Verification items for the finished model (mm, model axes). Round coordinates to 2 decimals unless told otherwise and drop trailing zeros. Write each loop counter-clockwise with the first axis right and the second up, starting at its lowest first coordinate (ties: lowest second). Pieces come first, ordered by that corner, then holes. Notation, with made-up numbers: (22.25, 75.5) - (77.25, 75.5) arc R26 cw to (77.25, 112.5) - close; hole circle Ø7 at (45.25, -25). An arc over 180 degrees is marked (long way). Answer as a JSON object with one key per item and string values.
```python
from build123d import *

# Parameters (mm, degrees)
F0_R     = 7.5
F1_DEPTH = 11


# Not quite as in the source:
# - a feature of the source that left no trace in its solid (it failed there, or was rolled back) is left out


with BuildPart() as f1:
    # F0 (on Front) → F1 (new body)
    with BuildSketch(Plane.XZ):
        with BuildLine():
            ThreePointArc((6.9961100303, 104.7666666667), (0, 98), (-6.9961100303, 104.7666666667))
            ThreePointArc((-6.9961100303, 104.7666666667), (-105, 0), (-6.9961100303, -104.7666666667))
            ThreePointArc((-6.9961100303, -104.7666666667), (0, -98), (6.9961100303, -104.7666666667))
            ThreePointArc((6.9961100303, -104.7666666667), (105, 0), (6.9961100303, 104.7666666667))
        make_face()
        with Locations((-59.54553545, -60.6574744609)):
            Circle(F0_R, mode=Mode.SUBTRACT)
        with Locations((-22.7581460876, -81.8966836121)):
            Circle(F0_R, mode=Mode.SUBTRACT)
        with Locations((-82.3036815375, -21.2392091511)):
            Circle(F0_R, mode=Mode.SUBTRACT)
        with Locations((22.7581460876, -81.8966836121)):
            Circle(F0_R, mode=Mode.SUBTRACT)
        with Locations((59.54553545, -60.6574744609)):
            Circle(F0_R, mode=Mode.SUBTRACT)
        with Locations((82.3036815375, -21.2392091511)):
            Circle(F0_R, mode=Mode.SUBTRACT)
        with Locations((-82.3036815375, 21.2392091511)):
            Circle(F0_R, mode=Mode.SUBTRACT)
        with Locations((-59.54553545, 60.6574744609)):
            Circle(F0_R, mode=Mode.SUBTRACT)
        with BuildLine():
            ThreePointArc((-15.2581460876, 81.8966836121), (-16.7869427812, 77.3585418036), (-20.750074374, 74.6705056463))
            ThreePointArc((-20.750074374, 74.6705056463), (-28.729349394, 86.4348254206), (-15.2581460876, 81.8966836121))
        make_face(mode=Mode.SUBTRACT)
        with BuildLine():
            ThreePointArc((10.3081014632, 37.0943802243), (30.6521769727, 23.2957946169), (38.5, 0))
            ThreePointArc((38.5, 0), (-23.2957946169, -30.6521769727), (-10.3081014632, 37.0943802243))
            ThreePointArc((-10.3081014632, 37.0943802243), (0, 38.5), (10.3081014632, 37.0943802243))
        make_face(mode=Mode.SUBTRACT)
        with Locations((82.3036815375, 21.2392091511)):
            Circle(F0_R, mode=Mode.SUBTRACT)
        with BuildLine():
            ThreePointArc((30.2581460876, 81.8966836121), (27.2962878961, 75.9254803057), (20.750074374, 74.6705056463))
            ThreePointArc((20.750074374, 74.6705056463), (18.2200042791, 87.8678869184), (30.2581460876, 81.8966836121))
        make_face(mode=Mode.SUBTRACT)
        with Locations((59.54553545, 60.6574744609)):
            Circle(F0_R, mode=Mode.SUBTRACT)
    extrude(amount=F1_DEPTH)


solid = f1.part
```
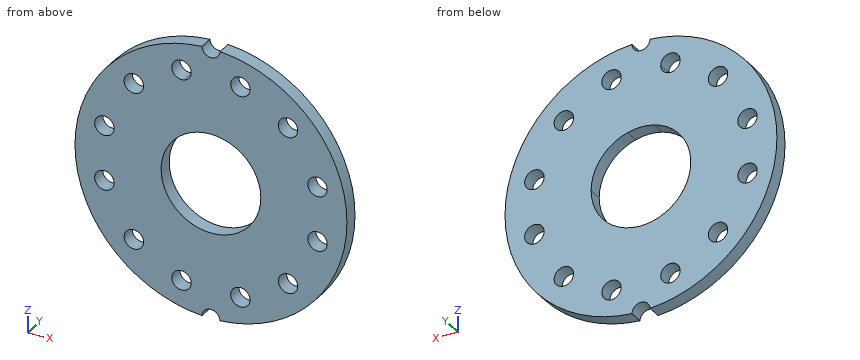
1. Material ranges on probe 1 along X at (y, z) = (-1.5, -20); probe 2 along X at (y, z) = (-4.25, -83.5); probe 3 along Z at (x, y) = (76, -4.25), recorded low to high. Write a range as from..to.
Completed:
{"probe 1": "x = -103.08..-89.7, -74.91..-32.9, 32.9..74.91, 89.7..103.08", "probe 2": "x = -63.66..-30.08, -15.43..15.43, 30.08..63.66", "probe 3": "z = -72.45..-25.3, -17.18..17.18, 25.3..72.45"}
2. Cross-section at D-D (y = -5). Count the separate pieces of the cut face and the enclosed holes in it, plus the area to 3 significant figures.
Completed:
{"separate pieces": "1", "enclosed holes": "13", "area": "27,700 mm^2"}
3. Cross-section at C-C (x = 0). Record the boundary of the cut face in (y, z), plus the area to 3 significant figures.
Completed:
{"outline": "(-11, -98) - (0, -98) - (0, -38.5) - (-11, -38.5) - close; (-11, 38.5) - (0, 38.5) - (0, 98) - (-11, 98) - close", "area": "1,310 mm^2"}
4. Go/stop test with flat-tipped pins: pin 1 (1 mm diameter, centred on y = -5, z = 4.5, fed in from +X); pin 2 (1 mm diameter, centred on y = -4.5, z = 56.5, fed in from -X); pin 3 (6 mm diameter, centred on y = -8, z = -29.5, fed in from +X). Record where each tip stops, or that it passes through.
Completed:
{"pin 1": "stops at x = 104.92", "pin 2": "stops at x = -88.82", "pin 3": "stops at x = 101.6"}
5. Cross-section at B-B (z = 32). Record the boundary of the cut face in (x, y) (3 decimals), plus the area to 3 significant figures.
Completed:
{"outline": "(-100.005, -11) - (-21.407, -11) - (-21.407, 0) - (-100.005, 0) - close; (21.407, -11) - (100.005, -11) - (100.005, 0) - (21.407, 0) - close", "area": "1,730 mm^2"}
6. Cross-section at A-A (x = 62). Record the boundary of the cut face in (y, z).
Completed:
{"outline": "(-11, -84.74) - (0, -84.74) - (0, -67.74) - (-11, -67.74) - close; (-11, -53.57) - (0, -53.57) - (0, 53.57) - (-11, 53.57) - close; (-11, 67.74) - (0, 67.74) - (0, 84.74) - (-11, 84.74) - close"}
